from build123d import *

# Parameters (mm, degrees)
BOSS_EXTRU_1_DEPTH = 5
CONG_1_R           = 40


with BuildPart() as part:
    # Esquisse1 → Boss.-Extru.1 (new body)
    with BuildSketch(Plane.XY):
        Polygon((0, 25), (0, 10), (-5, 10), (-5, 5), (0, 5), (0, 1.5), (3, 1.5), (3, 2.6), (5.3, 2.6), (5.3, 1.5), (10, 1.5), (10, -1.5), (5.3, -1.5), (5.3, -2.6), (3, -2.6), (3, -1.5), (0, -1.5), (0, -5), (-5, -5), (-5, -10), (0, -10), (0, -15), (55, -15), (55, 25), (50, 25), (50, 30), (45, 30), (45, 25), (41.5, 25), (41.5, 22), (42.6, 22), (42.6, 19.7), (41.5, 19.7), (41.5, 15), (38.5, 15), (38.5, 19.7), (37.4, 19.7), (37.4, 22), (38.5, 22), (38.5, 25), (35, 25), (35, 30), (30, 30), (30, 25), (25, 25), (25, 30), (20, 30), (20, 25), (16.5, 25), (16.5, 22), (17.6, 22), (17.6, 19.7), (16.5, 19.7), (16.5, 15), (13.5, 15), (13.5, 19.7), (12.4, 19.7), (12.4, 22), (13.5, 22), (13.5, 25), (10, 25), (10, 30), (5, 30), (5, 25), align=None)
    extrude(amount=BOSS_EXTRU_1_DEPTH)

    # Congé1
    cong_1_edges = [part.edges().sort_by_distance(p)[0] for p in [
        (55, -15, 2.5),
    ]]
    fillet(cong_1_edges, radius=CONG_1_R - 0.0001)  # a hair under: the kernel refuses the full size


solid = part.part
Here's how the part is built. I have some questions about the finished solid (model axes, mm). A direction names the side the tool comes from. Coordinates: 2 decimals unless noted, no trailing zeros. Write each loop counter-clockwise with the first axis right and the second up, starting at its lowest first coordinate (ties: lowest second). Pieces come first, ordered by that corner, then holes. Notation, with made-up numbers: (10.25, -34) - (56.25, -34) arc R22 cw to (56.25, -26) - close; hole circle Ø5 at (54, -20.5). An arc over 180 degrees is marked (long way). Use one line per item in the form item = value.
1) Suppose I cut it at B-B, the plane y = 8.5. Write out the boundary of the cut face in (x, z).
Solved:
outline = (-5, 0) - (51.44, 0) - (51.44, 5) - (-5, 5) - close
2) I'm going to push flat-ended pins straight in: P1, Ø2.5, axis at y = -0.5, z = 2.5, coming from the -X side; P2, Ø2.5, axis at x = 28, z = 2.5, coming from the +Y side; P3, Ø2, axis at y = 9, z = 3, coming from the +X side. Where does each tip first touch, or does it pass through?
Solved:
P1 = 0
P2 = 25
P3 = 52.08
3) Suppose I cut it at C-C, the plane x = 31.5. Write out the boundary of the cut face in (y, z), plus the area to 3 significant figures.
Solved:
outline = (-11.44, 0) - (30, 0) - (30, 5) - (-11.44, 5) - close
area = 207 mm2
4) I need wall thicknesses on line 1 (X direction, y = 26.5, z = 2.95); line 2 (X direction, y = 22.5, z = 2.15); line 3 (X direction, y = -7, z = 4.15). Which ranges of each line are inside material? Lowest first, please.
Solved:
line_1 = 5 to 10, 20 to 25, 30 to 35, 45 to 50
line_2 = 0 to 13.5, 16.5 to 38.5, 41.5 to 54.92
line_3 = -5 to 39
5) Suppose I cut it at A-A, the plane y = 23. Write out the boundary of the cut face in (x, z), plus the area to 3 significant figures.
Solved:
outline = (0, 0) - (13.5, 0) - (13.5, 5) - (0, 5) - close; (16.5, 0) - (38.5, 0) - (38.5, 5) - (16.5, 5) - close; (41.5, 0) - (54.95, 0) - (54.95, 5) - (41.5, 5) - close
area = 245 mm2
6) Thinking about a two-plate mould opening in Y: for faces 4 (the flat face through (42.6, 21, 2)), 5 (the flat face through (23, 30, 2)), 6 (the flat face through (8, -1.5, 2)), 7 (the flat face through (7, -15, 2)), which applies, released by +Y, released by -Y, zero draft, split by the parting line, or undercut?
Solved:
face_4 = undercut
face_5 = released by +Y
face_6 = undercut
face_7 = released by -Y
7) On a 3-axis mill with a long thin cutter (end or side, diameter ignored), from which of +Z, -Z, +X, -X, +Y, -Y can I reach the whole of each face in a straight line? I mean faces 1 (the flat face through (0, 18, 2)), 2 (the flat face through (40, 15, 2)), 3 (the flat face through (0, 3, 2)). Say none if no direction works.
Solved:
face_1 = +Z, -Z, -X, +Y
face_2 = +Z, -Z, +Y
face_3 = +Z, -Z, -X
